```python
from build123d import *

# Parameters (mm, degrees)
ESBO_O2_W                = 20
ESBO_O2_H                = 500
RESSALTO_EXTRUS_O1_DEPTH = 700
ESBO_O3_W                = 93.65
ESBO_O3_H                = 56.193
RESSALTO_EXTRUS_O2_DEPTH = 5
ESBO_O5_W                = 93.65
ESBO_O5_H                = 56.193
RESSALTO_EXTRUS_O3_DEPTH = 10
RESSALTO_EXTRUS_O4_DEPTH = 20
CORTE_EXTRUS_O1_DEPTH    = 116
FILETE1_R                = 10
ESBO_O8_W                = 3
ESBO_O8_H                = 10
RESSALTO_EXTRUS_O5_DEPTH = 8
FILETE2_R                = 3
ESBO_O9_R                = 1.5
CORTE_EXTRUS_O2_DEPTH    = 8
ESPELHAR1_START          = 5
ESPELHAR1_OUTLINE_R      = 1.5
ESPELHAR1_DEPTH          = 5
ESPELHAR1_START_2        = 10
ESPELHAR1_2_OUTLINE_R    = 1.5
ESPELHAR1_2_DEPTH        = 3
ESBO_O12_W               = 10
ESBO_O12_H               = 3
RESSALTO_EXTRUS_O6_DEPTH = 8
FILETE3_R                = 3
ESBO_O13_R               = 1.5
CORTE_EXTRUS_O3_DEPTH    = 8


# Read off the part's stored shape, not the designer's step: Espelhar1
with BuildPart() as part:
    # Esboço2 → Ressalto-extrusão1 (new body)
    with BuildSketch(Plane(origin=(0, 0, 0), x_dir=(0, 0, -1), z_dir=(1, 0, 0))):
        with Locations((10, 250)):
            Rectangle(ESBO_O2_W, ESBO_O2_H)
    extrude(amount=RESSALTO_EXTRUS_O1_DEPTH)

    # Esboço3 → Ressalto-extrusão2 (add)
    with BuildSketch(Plane.XY):
        with Locations((350, 250)):
            Rectangle(ESBO_O3_W, ESBO_O3_H)
    extrude(amount=RESSALTO_EXTRUS_O2_DEPTH)

    # Esboço5 → Ressalto-extrusão3 (add)
    with BuildSketch(Plane.XY):
        with BuildLine():
            Line((293.175, 191.9035), (406.825, 191.9035))
            ThreePointArc((406.825, 191.9035), (420.967135624, 197.761364376), (426.825, 211.9035))
            Line((426.825, 211.9035), (426.825, 288.0965))
            ThreePointArc((426.825, 288.0965), (420.967135624, 302.238635624), (406.825, 308.0965))
            Line((406.825, 308.0965), (293.175, 308.0965))
            ThreePointArc((293.175, 308.0965), (279.032864376, 302.238635624), (273.175, 288.0965))
            Line((273.175, 288.0965), (273.175, 211.9035))
            ThreePointArc((273.175, 211.9035), (279.032864376, 197.761364376), (293.175, 191.9035))
        make_face()
        with Locations((350, 250)):
            Rectangle(ESBO_O5_W, ESBO_O5_H, mode=Mode.SUBTRACT)
    extrude(amount=RESSALTO_EXTRUS_O3_DEPTH)

    # Esboço6 → Ressalto-extrusão4 (add)
    with BuildSketch(Plane.XY.offset(10)):
        with BuildLine():
            Line((298.175, 241.0965), (298.175, 278.0965))
            ThreePointArc((298.175, 278.0965), (299.639466094, 281.632033906), (303.175, 283.0965))
            Line((303.175, 283.0965), (396.825, 283.0965))
            ThreePointArc((396.825, 283.0965), (400.360533906, 281.632033906), (401.825, 278.0965))
            Line((401.825, 278.0965), (401.825, 241.0965))
            Line((401.825, 241.0965), (404.825, 241.0965))
            Line((404.825, 241.0965), (404.825, 281.0965))
            ThreePointArc((404.825, 281.0965), (403.360533906, 284.632033906), (399.825, 286.0965))
            Line((399.825, 286.0965), (300.175, 286.0965))
            ThreePointArc((300.175, 286.0965), (296.639466094, 284.632033906), (295.175, 281.0965))
            Line((295.175, 281.0965), (295.175, 241.0965))
            Line((295.175, 241.0965), (298.175, 241.0965))
        make_face()
    extrude(amount=RESSALTO_EXTRUS_O4_DEPTH)

    # Esboço7 → Corte-extrusão1 (cut)
    with BuildSketch(Plane(origin=(404.825, 0, 0), x_dir=(0, 0, -1), z_dir=(1, 0, 0))):
        Polygon((-10, 241.0965), (-30, 261.0965), (-30, 241.0965), align=None)
    extrude(amount=-CORTE_EXTRUS_O1_DEPTH, mode=Mode.SUBTRACT)

    # Filete1
    filete1_edges = [part.edges().sort_by_distance(p)[0] for p in [
        (403.325, 261.0965, 30),
        (296.675, 261.0965, 30),
    ]]
    fillet(filete1_edges, radius=FILETE1_R)

    # Esboço8 → Ressalto-extrusão5 (add)
    with BuildSketch(Plane.ZY.offset(-295.175)):
        with Locations((11.5, 263.5965)):
            Rectangle(ESBO_O8_W, ESBO_O8_H)
    extrude(amount=RESSALTO_EXTRUS_O5_DEPTH)

    # Filete2
    filete2_edges = [part.edges().sort_by_distance(p)[0] for p in [
        (295.175, 258.5965, 11.5),
        (295.175, 268.5965, 11.5),
        (287.175, 258.5965, 11.5),
        (287.175, 268.5965, 11.5),
    ]]
    fillet(filete2_edges, radius=FILETE2_R)

    # Esboço9 → Corte-extrusão2 (cut)
    with BuildSketch(Plane.XY.offset(13)):
        with Locations((291.175, 263.5965)):
            Circle(ESBO_O9_R)
    extrude(amount=-CORTE_EXTRUS_O2_DEPTH, mode=Mode.SUBTRACT)

    # Espelhar1 outline → Espelhar1 (cut)
    with BuildSketch(Plane.XY.offset(ESPELHAR1_START)):
        with Locations((408.825, 263.5965)):
            Circle(ESPELHAR1_OUTLINE_R)
    extrude(amount=ESPELHAR1_DEPTH, mode=Mode.SUBTRACT)

    # Espelhar1 2 outline → Espelhar1 2 (add)
    with BuildSketch(Plane.XY.offset(ESPELHAR1_START_2)):
        with BuildLine():
            Line((404.825, 268.5965), (404.825, 258.5965))
            Line((404.825, 258.5965), (409.825, 258.5965))
            ThreePointArc((409.825, 258.5965), (411.946320344, 259.475179656), (412.825, 261.5965))
            Line((412.825, 261.5965), (412.825, 265.5965))
            ThreePointArc((412.825, 265.5965), (411.946320344, 267.717820344), (409.825, 268.5965))
            Line((409.825, 268.5965), (404.825, 268.5965))
        make_face()
        with Locations((408.825, 263.5965)):
            Circle(ESPELHAR1_2_OUTLINE_R, mode=Mode.SUBTRACT)
    extrude(amount=ESPELHAR1_2_DEPTH)

    # Esboço12 → Ressalto-extrusão6 (add)
    with BuildSketch(Plane(origin=(0, 286.0965, 0), x_dir=(1, 0, 0), z_dir=(0, 1, 0))):
        with Locations((350, -11.5)):
            Rectangle(ESBO_O12_W, ESBO_O12_H)
    extrude(amount=RESSALTO_EXTRUS_O6_DEPTH)

    # Filete3
    filete3_edges = [part.edges().sort_by_distance(p)[0] for p in [
        (355, 286.0965, 11.5),
        (345, 286.0965, 11.5),
        (355, 294.0965, 11.5),
        (345, 294.0965, 11.5),
    ]]
    fillet(filete3_edges, radius=FILETE3_R)

    # Esboço13 → Corte-extrusão3 (cut)
    with BuildSketch(Plane.XY.offset(13)):
        with Locations((350, 290.0965)):
            Circle(ESBO_O13_R)
    extrude(amount=-CORTE_EXTRUS_O3_DEPTH, mode=Mode.SUBTRACT)


solid = part.part
```
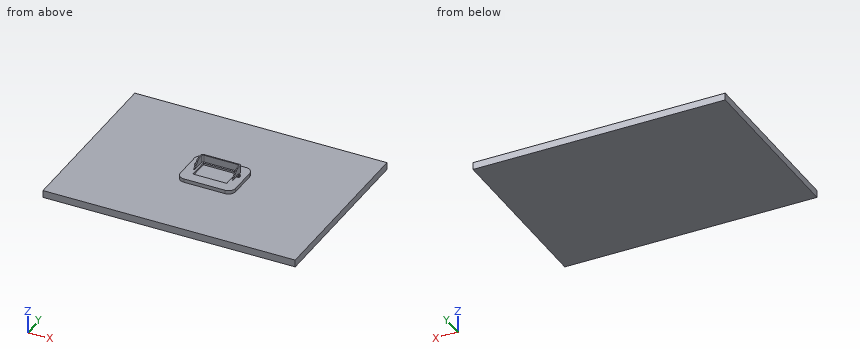
Work out the finished part from the listing and answer in its coordinate system (mm). Coordinates: 2 decimals unless noted, no trailing zeros. Loops run counter-clockwise (first coordinate to the right, second up) from the corner with the lowest first, then second, coordinate; pieces in that order, holes last. Notation, with made-up numbers: (-3, 63) - (44, 63) arc R10 ccw to (44, 68) - close; hole circle Ø8 at (52, 58.25). An arc over 180 degrees is marked (long way). Use a Markdown table: item, result.
Item 1: Find section B-B, the plane x = 523.5. Determine the outline of the cut face in (y, z).
Evaluation:
| item | result |
|---|---|
| outline | (0, -20) - (500, -20) - (500, 0) - (0, 0) - close |
Item 2: Find section A-A, the plane y = 94. Determine the outline of the cut face in (x, z).
Evaluation:
| item | result |
|---|---|
| outline | (0, -20) - (700, -20) - (700, 0) - (0, 0) - close |
Item 3: Consider probe 1 along Y at (x, z) = (350, 6.5); probe 2 along Y at (x, z) = (391, 9); probe 3 along Z at (x, y) = (603.5, 422). Determine where each line is inside the solid, lowest interval first. Write a range as from..to.
Evaluation:
| item | result |
|---|---|
| probe 1 | y = 191.9..221.9, 278.1..288.6, 291.6..308.1 |
| probe 2 | y = 191.9..221.9, 278.1..308.1 |
| probe 3 | z = -20..0 |
Item 4: Given pin 1 Ø4 at (x, y) = (410, 263) entering from +Z; pin 2 Ø2 at (x, y) = (303.5, 319.5) entering from +Z; pin 3 Ø2.5 at (x, z) = (360, 7.5) entering from -Y, each flat-ended and moving along its own axis, determine where each tip first touches the part or whether it passes through.
Evaluation:
| item | result |
|---|---|
| pin 1 | stops at z = 13 |
| pin 2 | stops at z = 0 |
| pin 3 | stops at y = 191.9 |
